Design review of the part built by this model. Coordinates are the model's own, in mm. A direction names the side the tool comes from. Give positions to 0.01 mm unless a question says otherwise; leave off trailing zeros. Loops run counter-clockwise (first coordinate to the right, second up) from the corner with the lowest first, then second, coordinate; pieces in that order, holes last. Notation, with made-up numbers: (-22, 58) - (11, 58) arc R20 ccw to (11, 63) - close; hole circle Ø10 at (9, 27.25). An arc over 180 degrees is marked (long way). Write each question's results on one line, items separated by ' | '.
from build123d import *

# Parameters (mm, degrees)
SKETCH2_R           = 2.475
BOSS_EXTRUDE1_DEPTH = 37.5
CIRPATTERN1_COUNT   = 2
CIRPATTERN1_ANGLE   = 90


with BuildPart() as part:
    # Sketch2 → Boss-Extrude1 (new, symmetric)
    with BuildSketch(Plane.XY):
        Circle(SKETCH2_R)
    boss_extrude1 = extrude(amount=BOSS_EXTRUDE1_DEPTH, both=True)

    # CirPattern1: Boss-Extrude1 ×2 about axis
    cirpattern1_axis = Axis((0, -2.7225, 0), (0, 1, 0))
    for i in range(1, CIRPATTERN1_COUNT):
        add(boss_extrude1.rotate(cirpattern1_axis, i * CIRPATTERN1_ANGLE / (CIRPATTERN1_COUNT - 1)))


solid = part.part
(1) Wall thickness on line 1 along Z through (x, y) = (31.5, 0.2); line 2 along X through (y, z) = (-1.75, -13): over which ranges is each line inside the solid? List them lowest first. Write a range as from..to.
Answers below:
line 1: -2.47..2.47 | line 2: -1.75..1.75
(2) Tool access review of faces 1 (the cylindrical face through (2.286, -0.948, -18.488)), 2 (the flat face through (0, 0, 37.5)), 3 (the cylindrical face through (-18.49, 0.74, -2.36)), 4 (the cylindrical face through (-0.537, -2.416, 19.012)), 5 (the cylindrical face through (19.012, -2.416, 0.537)): name each direction out of +Z, -Z, +X, -X, +Y, -Y from which nothing blocks a thin tool from reaching the whole face with its end or side.
Answers below:
face 1: -Z | face 2: +Z, +X, -X, +Y, -Y | face 3: -X | face 4: +Z | face 5: +X
(3) Insertion check: P1, Ø2, axis at y = -1, z = 23.5, coming from the +X side (3 decimals); P2, Ø1, axis at x = -24, y = 1, coming from the +Z side; P3, Ø8, axis at x = 8, z = -8, coming from the -Y side. Each pin has a flat end and moves straight along its axis. Give the tip position at first contact, or say it passes through.
Answers below:
P1: x = 2.475 | P2: z = 2.42 | P3: through
(4) Take a section at A-A on y = 0. Give the boundary of the cut face in (x, z) (3 decimals).
Answers below:
outline: (-37.5, -2.475) - (-2.475, -2.475) - (-2.475, -37.5) - (2.475, -37.5) - (2.475, -2.475) - (37.5, -2.475) - (37.5, 2.475) - (2.475, 2.475) - (2.475, 37.5) - (-2.475, 37.5) - (-2.475, 2.475) - (-37.5, 2.475) - close
(5) Take a section at B-B on z = 16. Give the boundary of the cut face in (x, y) (3 decimals), plus the area to 3 significant figures.
Answers below:
outline: circle Ø4.95 at (0, 0) | area: 19.2 mm2
